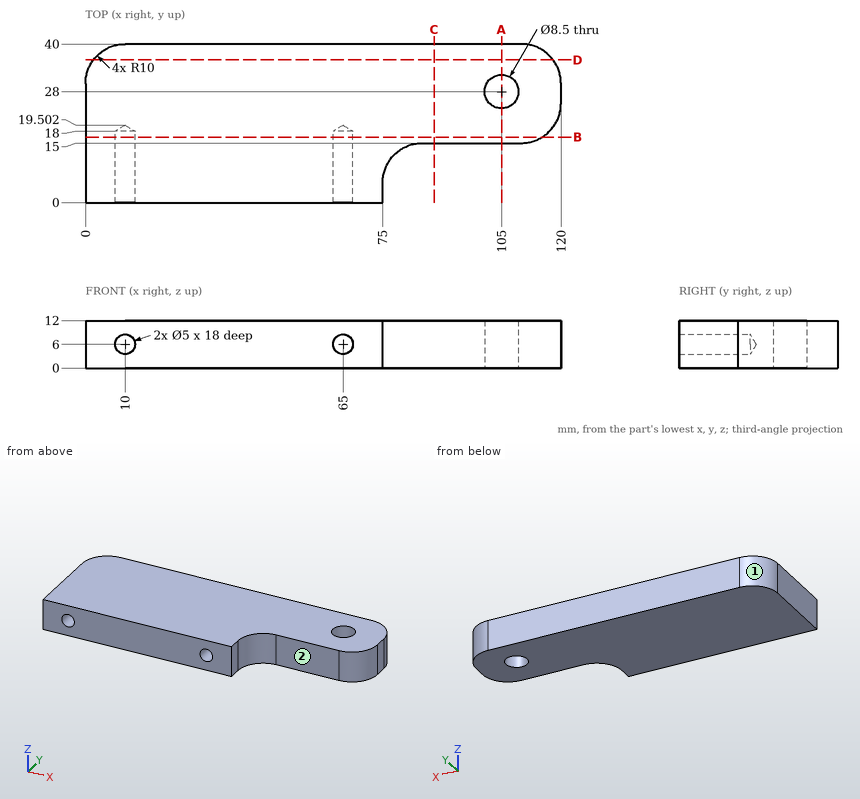
Verification items for this drawing (mm, ordinates from the low corner). A direction names the side the tool comes from. Coordinates: 2 decimals unless noted, no trailing zeros. Loops run counter-clockwise (first coordinate to the right, second up) from the corner with the lowest first, then second, coordinate; pieces in that order, holes last. Notation, with made-up numbers: (63, 59.25) - (96, 59.25) arc R16 ccw to (96, 81.25) - close; hole circle Ø4 at (38.25, 83). An arc over 180 degrees is marked (long way). One line per item, written item: value. Start each with the question number.
(1) Cross-section at C-C on x = 88. Enter the section's corners in (y, z).
(2) Tool access check on the marked faces 1 and 2. Record the directions out of +Z, -Z, +X, -X, +Y, -Y that give a thin tool (end or side, any length) a straight path to the whole face; none if there is none.
(3) Cross-section at D-D on y = 36. Enter the section's corners in (x, z).
(4) Depth check by flat-ended pin: P1, Ø3, axis at x = 65, z = 6, coming from the -Y side; P2, Ø5, axis at x = 105, y = 28, coming from the +Z side; P3, Ø2.5, axis at y = 2.5, z = 4, coming from the +X side; P4, Ø6, axis at x = 93.5, z = 7, coming from the -Y side. Enter the tip coordinate at first touch or a pass-through.
(5) Cross-section at A-A on x = 105. Enter the section's corners in (y, z).
(6) Material ranges on line 1 (Z direction, x = 10, y = 5.75); line 2 (Y direction, x = 105, z = 3); line 3 (X direction, y = 26.5, z = 4), recorded low to high. Write a range as [from, to].
(7) Cross-section at B-B on y = 16.5. Enter the section's corners in (x, z).
Results below:
1. outline: (15, 0) - (40, 0) - (40, 12) - (15, 12) - close
2. face 1: +Z, -Z, -X, +Y
2. face 2: +Z, -Z, +X, -Y
3. outline: (2, 0) - (118, 0) - (118, 12) - (2, 12) - close
4. P1: stops at y = 18.6
4. P2: passes through
4. P3: stops at x = 75
4. P4: stops at y = 15
5. outline: (15, 0) - (23.75, 0) - (23.75, 12) - (15, 12) - close; (32.25, 0) - (40, 0) - (40, 12) - (32.25, 12) - close
6. line 1: z = [0, 3.5], [8.5, 12]
6. line 2: y = [15, 23.75], [32.25, 40]
6. line 3: x = [0, 101.02], [108.98, 120]
7. outline: (0, 0) - (115.27, 0) - (115.27, 12) - (0, 12) - close; hole circle Ø5 at (10, 6); hole circle Ø5 at (65, 6)
